Model file for the job. Use its own axes, mm. Coordinates: 2 decimals unless noted, no trailing zeros. Write each loop counter-clockwise with the first axis right and the second up, starting at its lowest first coordinate (ties: lowest second). Pieces come first, ordered by that corner, then holes.
Q1. Band-saw the part on B-B, the plane z = 14.25. Write the cut outline in (x, y), plus the area to 3 significant figures.
Q2. Band-saw the part on A-A, the plane y = 92.5. Write the cut outline in (x, z), plus the area to 3 significant figures.
Q3. Drill centre lines: probe 1 along Y at (x, z) = (300, 14.5); probe 2 along X at (y, z) = (98, 10.25). Where is each one in solid material? Low to high.
Q4. Pin check, flat tips, straight feed: P1, Ø4, axis at y = 198, z = 12.5, coming from the -X side; P2, Ø1.5, axis at y = 340, z = 13, coming from the +X side; P3, Ø2.5, axis at x = 395, z = 12, coming from the +Y side. Stop position of each tip, or through.
from build123d import *

# Parameters (mm, degrees)
F0_W     = 564
F0_H     = 394
F1_DEPTH = 18
F0_W_2   = 18
F0_H_2   = 6
F2_DEPTH = 9


with BuildPart() as f1:
    # F0 (on Top) → F1 (new body)
    with BuildSketch(Plane.XY):
        with Locations((300, 197)):
            Rectangle(F0_W, F0_H)
    extrude(amount=F1_DEPTH)

    # F0 (on Top) → F2 (join)
    with BuildSketch(Plane.XY):
        with Locations((9, 197)):
            Rectangle(F0_W_2, F0_H)
        with Locations((300, 397)):
            Rectangle(F0_W, F0_H_2)
        with Locations((9, 397)):
            Rectangle(F0_W_2, F0_H_2)
        with Locations((591, 397)):
            Rectangle(F0_W_2, F0_H_2)
        with Locations((591, 197)):
            Rectangle(F0_W_2, F0_H)
    extrude(amount=F2_DEPTH)


solid = f1.part
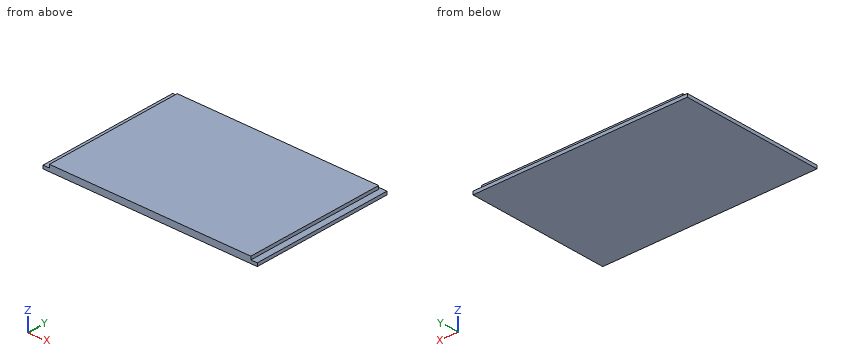
Answer sheet:
1. outline: (18, 0) - (582, 0) - (582, 394) - (18, 394) - close
1. area: 222,000 mm2
2. outline: (0, 0) - (600, 0) - (600, 9) - (582, 9) - (582, 18) - (18, 18) - (18, 9) - (0, 9) - close
2. area: 10,500 mm2
3. probe 1: y = 0 to 394
3. probe 2: x = 18 to 582
4. P1: stops at x = 18
4. P2: stops at x = 582
4. P3: stops at y = 394
